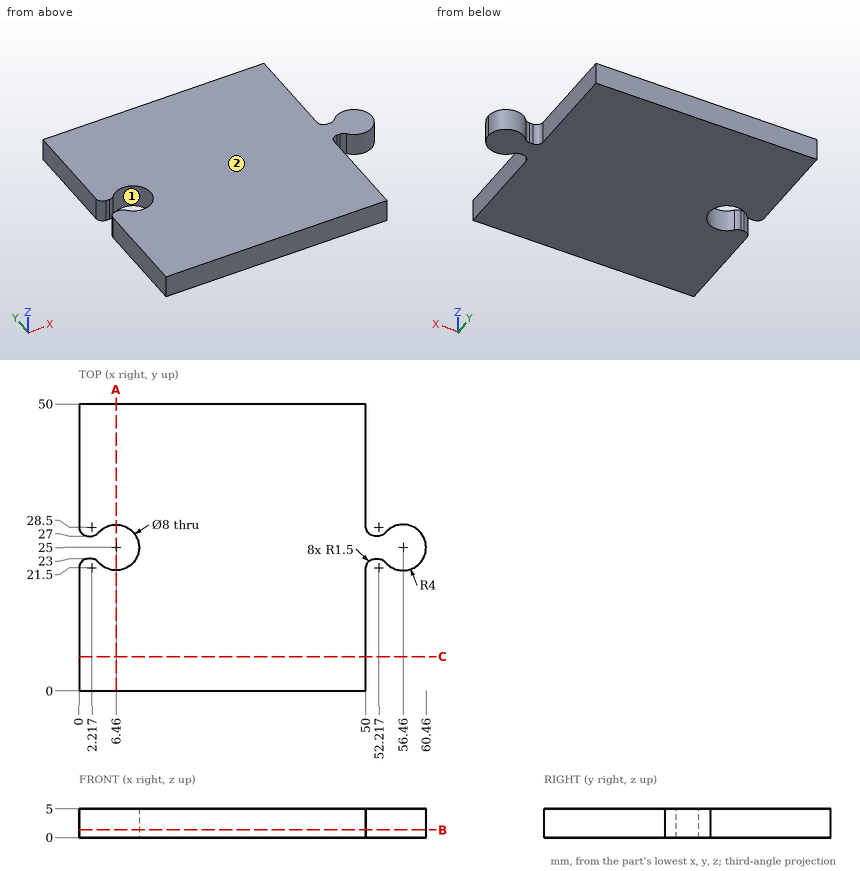
Verification items for this drawing (mm, ordinates from the low corner). Give positions to 0.01 mm unless a question says otherwise; leave off trailing zeros. Order: outer loops, then holes, each group sorted by start corner. A loop starts at its lowest first (then second) coordinate and runs counter-clockwise, first axis right, second up.
1) Cross-section at B-B (z = 1.35). Record the boundary of the cut face in (x, y) (1 decimal).
Results are:
outline: (0, 0) - (50, 0) - (50, 21.5) arc R1.5 cw to (51.5, 23) - (52.2, 23) arc R1.5 cw to (53.4, 22.5) arc R4 ccw (long way) to (53.4, 27.5) arc R1.5 cw to (52.2, 27) - (51.5, 27) arc R1.5 cw to (50, 28.5) - (50, 50) - (0, 50) - (0, 28.5) arc R1.5 ccw to (1.5, 27) - (2.2, 27) arc R1.5 ccw to (3.4, 27.5) arc R4 cw (long way) to (3.4, 22.5) arc R1.5 ccw to (2.2, 23) - (1.5, 23) arc R1.5 ccw to (0, 21.5) - close
2) Cross-section at C-C (y = 6). Record the boundary of the cut face in (x, z).
Results are:
outline: (0, 0) - (50, 0) - (50, 5) - (0, 5) - close
3) Material ranges on probe 1 along Y at (x, z) = (6.46, 2.95); probe 2 along X at (y, z) = (8.5, 1.5); probe 3 along X at (y, z) = (22, 0.3) (1 decimal), recorded low to high.
Results are:
probe 1: y = 0 to 21, 29 to 50
probe 2: x = 0 to 50
probe 3: x = 0.1 to 3.8, 9.1 to 50.1, 53.8 to 59.1
4) Gauge pin test, flat ends, axial feed: pin 1 (0.8 mm diameter, centred on x = 2, z = 3, fed in from -Y); pin 2 (0.8 mm diameter, centred on x = 51.5, z = 2.5, fed in from -Y) (1 decimal); pin 3 (1.5 mm diameter, centred on y = 35.5, z = 3, fed in from +X). Record the tip position at first contact, or that the pin passes through.
Results are:
pin 1: stops at y = 0
pin 2: stops at y = 22.9
pin 3: stops at x = 50
5) Draft check along X on the marked faces 1 and 2. Enter one of: released by +X, released by -X, zero draft, split by the parting line, or undercut.
Results are:
face 1: undercut
face 2: zero draft
6) Cross-section at A-A (x = 6.46). Record the boundary of the cut face in (y, z), then the cut area to 3 significant figures.
Results are:
outline: (0, 0) - (21, 0) - (21, 5) - (0, 5) - close; (29, 0) - (50, 0) - (50, 5) - (29, 5) - close
area: 210 mm2
